Job drawing, mm, ordinate dimensions from the low corner. One solid piece. Round coordinates to 2 decimals unless told otherwise and drop trailing zeros. Order: outer loops, then holes, each group sorted by start corner. A loop starts at its lowest first (then second) coordinate and runs counter-clockwise, first axis right, second up. Notation, with made-up numbers: (-21.5, 27.5) -> (-10.5, 27.5) arc R31 ccw to (-10.5, 64.5) -> close; hole circle Ø2 at (55.25, 9). An arc over 180 degrees is marked (long way). Return JSON: item names as keys, results as strings. Group by question number.
Q1. Probe line 1 along Y through (x, z) = (557, 246.5). List the from-to ranges inside material, lowest first.
Q2. Cut at A-A (y = 88). Write the cut outline in (x, z).
Q3. Cut at C-C (x = 219). Write the cut outline in (y, z).
Q4. Flat gauge pin, fed straight in: pin 1 (4 mm diameter, centred on x = 115, z = 211.5, fed in from -Y). Where does the tip first touch, or does it go through?
Q5. Cut at B-B (z = 359). Write the cut outline in (x, y).
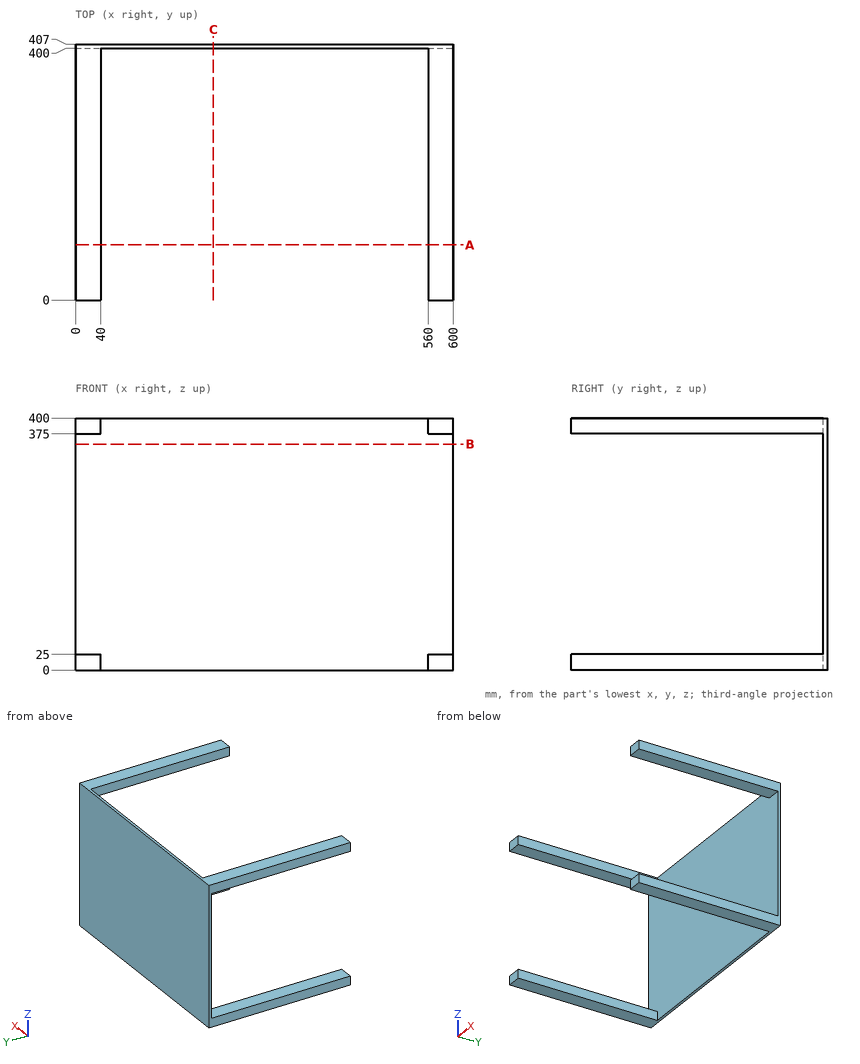
Solution:
{
 "1": {"line 1": "y = 400 to 407"},
 "2": {"outline": "(0, 0) -> (40, 0) -> (40, 25) -> (0, 25) -> close; (0, 375) -> (40, 375) -> (40, 400) -> (0, 400) -> close; (560, 0) -> (600, 0) -> (600, 25) -> (560, 25) -> close; (560, 375) -> (600, 375) -> (600, 400) -> (560, 400) -> close"},
 "3": {"outline": "(400, 0) -> (407, 0) -> (407, 400) -> (400, 400) -> close"},
 "4": {"pin 1": "stops at y = 400"},
 "5": {"outline": "(0, 400) -> (600, 400) -> (600, 407) -> (0, 407) -> close"}
}
